from build123d import *

# Parameters (mm, degrees)
DOME1_FACE_RADIUS   = 14.488501688
DOME1_HEIGHT        = 10
SKETCH4_W           = 2.198846944
SKETCH4_H           = 53.513980491
BOSS_EXTRUDE1_DEPTH = 96
SKETCH5_R           = 2.935842155
BOSS_EXTRUDE2_DEPTH = 114
SKETCH7_W           = 1.028080296
SKETCH7_H           = 31.194109998
BOSS_EXTRUDE3_DEPTH = 10


with BuildPart() as part:
    # Sketch1 → Revolve1 (revolve)
    with BuildSketch(Plane.XY):
        Polygon((0, 78.360347155), (-14.488501688, 78.360347155), (-14.488501688, 2.448760849), (-5.917838717, -6.121902122), (-5.917838717, -13.468184667), (-14.488501688, -13.468184667), (-14.488501688, -22.038847637), (-5.917838717, -22.038847637), (-5.917838717, -30.201383799), (-14.488501688, -30.201383799), (-14.488501688, -37.547666345), (-5.917838717, -37.547666345), (-5.917838717, -43.669568467), (-14.488501688, -43.669568467), (-14.488501688, -52.648358245), (-5.917838717, -52.648358245), (0, -52.648358245), align=None)
    revolve(axis=Axis((0, 93.052912247, 0), (0, -1, 0)))

    # Dome1: a dome of height H over a round flat face of radius A is a cap of a sphere of radius (A * A + H * H) / (2 * H)
    dome1_r = (DOME1_FACE_RADIUS * DOME1_FACE_RADIUS + DOME1_HEIGHT * DOME1_HEIGHT) / (2 * DOME1_HEIGHT)
    dome1_base = Plane((0, 78.360347155, 0), z_dir=(0, 1, 0))
    with Locations(dome1_base.offset(DOME1_HEIGHT - dome1_r)):
        dome1_ball = Sphere(dome1_r, mode=Mode.PRIVATE)
    add(split(dome1_ball, bisect_by=dome1_base, keep=Keep.TOP, mode=Mode.PRIVATE))

    # Sketch4 → Boss-Extrude1 (add)
    with BuildSketch(Plane.XY):
        with Locations((-4.762390363, 41.15200271)):
            Rectangle(SKETCH4_W, SKETCH4_H)
    boss_extrude1 = extrude(amount=BOSS_EXTRUDE1_DEPTH)

    # Mirror1: Boss-Extrude1 across plane
    add(boss_extrude1.mirror(Plane.XY))

    # Sketch5 → Boss-Extrude2 (add)
    with BuildSketch(Plane.XZ.offset(52.648358245)):
        Circle(SKETCH5_R)
    extrude(amount=BOSS_EXTRUDE2_DEPTH)

    # Sketch7 → Boss-Extrude3 (add)
    with BuildSketch(Plane.XZ.offset(166.648358245)):
        Rectangle(SKETCH7_W, SKETCH7_H)
    extrude(amount=BOSS_EXTRUDE3_DEPTH)


solid = part.part
The listing builds one solid part. Answer for the finished solid, in the listing's coordinates (mm). A direction names the side the tool comes from. Coordinates: 2 decimals unless noted, no trailing zeros. Order: outer loops, then holes, each group sorted by start corner. A loop starts at its lowest first (then second) coordinate and runs counter-clockwise, first axis right, second up. Notation, with made-up numbers: (34.25, 39) -> (86.25, 39) arc R31 cw to (86.25, 64) -> close; hole circle Ø7 at (-1, -24). An arc over 180 degrees is marked (long way). Answer in a Markdown table with one row per item. Add a question column.
Item 1: Which of the six approach directions +Z, -Z, +X, -X, +Y, -Y give full straight-line access (tool end or side, diameter ignored) to faces 3 (the face through (-5.862, 41, -54)), 4 (the face through (-6.2, -37.548, -0.2)), 5 (the face through (-5.862, 41, 54))?
Item 2: Determine the mould class of faces 1 (the face through (0.514, -172, 0)), 2 (the face through (1.283, -9.846, 5.777)) for opening direction Y: +Y half, -Y half, draft (parallel to the pull), parting line (faces both ways), or undercut.
Item 3: Find section D-D (y = -81). Write down the section's boundary in (x, z).
Item 4: Find the intervals of material crossed by L1, parallel to X at y = 44, z = 73.5; L2, parallel to Z at x = 0.5, y = -90.5; L3, parallel to Z at x = -2, y = -64, in increasing order. Write a range as from..to.
Item 5: Find section C-C (x = 9). State how many separate pieces and enclosed holes the cut face has, then the cut area to 3 significant figures.
Item 6: Find section A-A (y = 63). Write down the section's boundary in (x, z), then the cut area to 3 significant figures.
Item 7: Each of these flat-tipped pins is pushed along its axis until it touches: P1, Ø2.5, axis at x = -4.5, z = 50.5, coming from the -Y side (3 decimals); P2, Ø0.7, axis at x = -1.5, z = 1.5, coming from the -Y side; P3, Ø1.1, axis at x = -5, z = -36.5, coming from the +Y side; P4, Ø8, axis at x = -8.5, y = -137.5, coming from the +Z side. Where does it stop, or does it pass through?
Item 8: Find section B-B (z = -52). Write down the section's boundary in (x, y).
Result set:
| question | item | result |
|---|---|---|
| 1 | face 3 | -Z, -X, +Y, -Y |
| 1 | face 4 | none |
| 1 | face 5 | +Z, -X, +Y, -Y |
| 2 | face 1 | draft |
| 2 | face 2 | undercut |
| 3 | outline | circle Ø5.87 at (0, 0) |
| 4 | L1 | x = -5.86..-3.66 |
| 4 | L2 | z = -2.89..2.89 |
| 4 | L3 | z = -2.15..2.15 |
| 5 | separate pieces | 4 |
| 5 | enclosed holes | 0 |
| 5 | area | 2,480 mm² |
| 6 | outline | (-5.86, -96) -> (-3.66, -96) -> (-3.66, -14.02) arc R14.49 ccw (long way) to (-3.66, 14.02) -> (-3.66, 96) -> (-5.86, 96) -> (-5.86, 13.25) arc R14.49 ccw to (-5.86, -13.25) -> close |
| 6 | area | 1,020 mm² |
| 7 | P1 | stops at y = 14.395 |
| 7 | P2 | stops at y = -166.65 |
| 7 | P3 | stops at y = 67.91 |
| 7 | P4 | passes through |
| 8 | outline | (-5.86, 14.4) -> (-3.66, 14.4) -> (-3.66, 67.91) -> (-5.86, 67.91) -> close |
